from build123d import *

# Parameters (mm, degrees)
SKETCH1_W                     = 935.9
SKETCH1_H                     = 526.4
SKETCH1_R                     = 57.5
BASE_FLANGE1_DEPTH            = 0.7366
EDGE_FLANGE1_STRIP_W          = 4.4196
EDGE_FLANGE1_STRIP_H          = 0.7366
EDGE_FLANGE1_STRIP_CUT_DEPTH  = 935.9
EDGE_FLANGE1_DEPTH            = 935.9
EDGE_FLANGE2_STRIP_W          = 4.4196
EDGE_FLANGE2_STRIP_H          = 0.7366
EDGE_FLANGE2_STRIP_CUT_DEPTH  = 524.9268
EDGE_FLANGE2_DEPTH            = 524.9268
EDGE_FLANGE3_STRIP_W          = 4.4196
EDGE_FLANGE3_STRIP_H          = 0.7366
EDGE_FLANGE3_STRIP_CUT_DEPTH  = 934.4268
EDGE_FLANGE3_DEPTH            = 934.4268
EDGE_FLANGE4_STRIP_W          = 4.4196
EDGE_FLANGE4_STRIP_H          = 0.7366
EDGE_FLANGE4_STRIP_CUT_DEPTH  = 523.4536
EDGE_FLANGE4_DEPTH            = 523.4536
EDGE_FLANGE5_STRIP_W          = 4.4196
EDGE_FLANGE5_STRIP_H          = 0.7366
EDGE_FLANGE5_STRIP_CUT_DEPTH  = 874.0268
EDGE_FLANGE5_RELIEF_W         = 4.7879
EDGE_FLANGE5_RELIEF_H         = 0.3683
EDGE_FLANGE5_RELIEF_CUT_DEPTH = 0.7366
EDGE_FLANGE5_DEPTH            = 874.0268
EDGE_FLANGE6_STRIP_W          = 4.4196
EDGE_FLANGE6_STRIP_H          = 0.7366
EDGE_FLANGE6_STRIP_CUT_DEPTH  = 874.0268
EDGE_FLANGE6_RELIEF_W         = 4.7879
EDGE_FLANGE6_RELIEF_H         = 0.3683
EDGE_FLANGE6_RELIEF_CUT_DEPTH = 0.7366
EDGE_FLANGE6_DEPTH            = 874.0268
EDGE_FLANGE7_STRIP_W          = 4.4196
EDGE_FLANGE7_STRIP_H          = 0.7366
EDGE_FLANGE7_STRIP_CUT_DEPTH  = 523.4536
EDGE_FLANGE7_DEPTH            = 523.4536
EDGE_FLANGE8_STRIP_W          = 4.4196
EDGE_FLANGE8_STRIP_H          = 0.7366
EDGE_FLANGE8_STRIP_CUT_DEPTH  = 523.9902
EDGE_FLANGE8_RELIEF_W         = 4.7879
EDGE_FLANGE8_RELIEF_H         = 0.3683
EDGE_FLANGE8_RELIEF_CUT_DEPTH = 0.7366
EDGE_FLANGE8_DEPTH            = 523.9902


# Sheet-metal steps are written as plain solids
with BuildPart() as part:
    # Sketch1 → Base-Flange1 (new body)
    with BuildSketch(Plane(origin=(0, 0, 0), x_dir=(0, 0, -1), z_dir=(1, 0, 0))):
        Rectangle(SKETCH1_W, SKETCH1_H)
        Circle(SKETCH1_R, mode=Mode.SUBTRACT)
    extrude(amount=-BASE_FLANGE1_DEPTH)

    # Edge-Flange1 strip (across the edge) → Edge-Flange1 strip cut (cut)
    with BuildSketch(Plane(origin=(-0.7366, 263.2, 467.95), x_dir=(0, -1, 0), z_dir=(0, 0, -1))):
        with Locations((-0.7366, -0.3683)):
            Rectangle(EDGE_FLANGE1_STRIP_W, EDGE_FLANGE1_STRIP_H)
    extrude(amount=EDGE_FLANGE1_STRIP_CUT_DEPTH, mode=Mode.SUBTRACT)

    # Edge-Flange1 section (across the edge) → Edge-Flange1 (add)
    with BuildSketch(Plane(origin=(-0.7366, 263.2, 467.95), x_dir=(0, -1, 0), z_dir=(0, 0, -1))):
        with BuildLine():
            Line((0, 0.7366), (0, 29.2634))
            Line((0, 29.2634), (0.7366, 29.2634))
            Line((0.7366, 29.2634), (0.7366, 0.7366))
            ThreePointArc((0.7366, 0.7366), (0.952345145, 0.215745145), (1.4732, 0))
            Line((1.4732, 0), (1.4732, -0.7366))
            ThreePointArc((1.4732, -0.7366), (0.43149029, -0.30510971), (0, 0.7366))
        make_face()
    extrude(amount=EDGE_FLANGE1_DEPTH)

    # Edge-Flange2 strip (across the edge) → Edge-Flange2 strip cut (cut)
    with BuildSketch(Plane(origin=(-0.7366, -263.2, 467.95), x_dir=(0, 0, -1), z_dir=(0, 1, 0))):
        with Locations((-0.7366, -0.3683)):
            Rectangle(EDGE_FLANGE2_STRIP_W, EDGE_FLANGE2_STRIP_H)
    extrude(amount=EDGE_FLANGE2_STRIP_CUT_DEPTH, mode=Mode.SUBTRACT)

    # Edge-Flange2 section (across the edge) → Edge-Flange2 (add)
    with BuildSketch(Plane(origin=(-0.7366, -263.2, 467.95), x_dir=(0, 0, -1), z_dir=(0, 1, 0))):
        with BuildLine():
            Line((0, 0.7366), (0, 29.2634))
            Line((0, 29.2634), (0.7366, 29.2634))
            Line((0.7366, 29.2634), (0.7366, 0.7366))
            ThreePointArc((0.7366, 0.7366), (0.952345145, 0.215745145), (1.4732, 0))
            Line((1.4732, 0), (1.4732, -0.7366))
            ThreePointArc((1.4732, -0.7366), (0.43149029, -0.30510971), (0, 0.7366))
        make_face()
    extrude(amount=EDGE_FLANGE2_DEPTH)

    # Edge-Flange3 strip (across the edge) → Edge-Flange3 strip cut (cut)
    with BuildSketch(Plane(origin=(-0.7366, -263.2, -467.95), x_dir=(0, 1, 0), z_dir=(0, 0, 1))):
        with Locations((-0.7366, -0.3683)):
            Rectangle(EDGE_FLANGE3_STRIP_W, EDGE_FLANGE3_STRIP_H)
    extrude(amount=EDGE_FLANGE3_STRIP_CUT_DEPTH, mode=Mode.SUBTRACT)

    # Edge-Flange3 section (across the edge) → Edge-Flange3 (add)
    with BuildSketch(Plane(origin=(-0.7366, -263.2, -467.95), x_dir=(0, 1, 0), z_dir=(0, 0, 1))):
        with BuildLine():
            Line((0, 0.7366), (0, 29.2634))
            Line((0, 29.2634), (0.7366, 29.2634))
            Line((0.7366, 29.2634), (0.7366, 0.7366))
            ThreePointArc((0.7366, 0.7366), (0.952345145, 0.215745145), (1.4732, 0))
            Line((1.4732, 0), (1.4732, -0.7366))
            ThreePointArc((1.4732, -0.7366), (0.43149029, -0.30510971), (0, 0.7366))
        make_face()
    extrude(amount=EDGE_FLANGE3_DEPTH)

    # Edge-Flange4 strip (across the edge) → Edge-Flange4 strip cut (cut)
    with BuildSketch(Plane(origin=(-0.7366, 261.7268, -467.95), x_dir=(0, 0, 1), z_dir=(0, -1, 0))):
        with Locations((-0.7366, -0.3683)):
            Rectangle(EDGE_FLANGE4_STRIP_W, EDGE_FLANGE4_STRIP_H)
    extrude(amount=EDGE_FLANGE4_STRIP_CUT_DEPTH, mode=Mode.SUBTRACT)

    # Edge-Flange4 section (across the edge) → Edge-Flange4 (add)
    with BuildSketch(Plane(origin=(-0.7366, 261.7268, -467.95), x_dir=(0, 0, 1), z_dir=(0, -1, 0))):
        with BuildLine():
            Line((0, 0.7366), (0, 29.2634))
            Line((0, 29.2634), (0.7366, 29.2634))
            Line((0.7366, 29.2634), (0.7366, 0.7366))
            ThreePointArc((0.7366, 0.7366), (0.952345145, 0.215745145), (1.4732, 0))
            Line((1.4732, 0), (1.4732, -0.7366))
            ThreePointArc((1.4732, -0.7366), (0.43149029, -0.30510971), (0, 0.7366))
        make_face()
    extrude(amount=EDGE_FLANGE4_DEPTH)

    # Edge-Flange5 strip (across the edge) → Edge-Flange5 strip cut (cut)
    with BuildSketch(Plane(origin=(-30, 262.4634, 437.0134), x_dir=(1, 0, 0), z_dir=(0, 0, -1))):
        with Locations((-0.7366, -0.3683)):
            Rectangle(EDGE_FLANGE5_STRIP_W, EDGE_FLANGE5_STRIP_H)
    extrude(amount=EDGE_FLANGE5_STRIP_CUT_DEPTH, mode=Mode.SUBTRACT)

    # Edge-Flange5 relief (on the sheet) → Edge-Flange5 relief cut (cut)
    with BuildSketch(Plane(origin=(-28.5268, 262.4634, 437.0134), x_dir=(1, 0, 0), z_dir=(0, -1, 0))):
        with Locations((-2.02565, 0.18415)):
            Rectangle(EDGE_FLANGE5_RELIEF_W, EDGE_FLANGE5_RELIEF_H)
        with Locations((-2.02565, -874.21095)):
            Rectangle(EDGE_FLANGE5_RELIEF_W, EDGE_FLANGE5_RELIEF_H)
    extrude(amount=-EDGE_FLANGE5_RELIEF_CUT_DEPTH, mode=Mode.SUBTRACT)

    # Edge-Flange5 section (across the edge) → Edge-Flange5 (add)
    with BuildSketch(Plane(origin=(-30, 262.4634, 437.0134), x_dir=(1, 0, 0), z_dir=(0, 0, -1))):
        with BuildLine():
            Line((0, 0.7366), (0, 29.2634))
            Line((0, 29.2634), (0.7366, 29.2634))
            Line((0.7366, 29.2634), (0.7366, 0.7366))
            ThreePointArc((0.7366, 0.7366), (0.952345145, 0.215745145), (1.4732, 0))
            Line((1.4732, 0), (1.4732, -0.7366))
            ThreePointArc((1.4732, -0.7366), (0.43149029, -0.30510971), (0, 0.7366))
        make_face()
    extrude(amount=EDGE_FLANGE5_DEPTH)

    # Edge-Flange6 strip (across the edge) → Edge-Flange6 strip cut (cut)
    with BuildSketch(Plane(origin=(-30, -262.4634, -437.0134), x_dir=(1, 0, 0), z_dir=(0, 0, 1))):
        with Locations((-0.7366, -0.3683)):
            Rectangle(EDGE_FLANGE6_STRIP_W, EDGE_FLANGE6_STRIP_H)
    extrude(amount=EDGE_FLANGE6_STRIP_CUT_DEPTH, mode=Mode.SUBTRACT)

    # Edge-Flange6 relief (on the sheet) → Edge-Flange6 relief cut (cut)
    with BuildSketch(Plane(origin=(-28.5268, -262.4634, -437.0134), x_dir=(1, 0, 0), z_dir=(0, 1, 0))):
        with Locations((-2.02565, 0.18415)):
            Rectangle(EDGE_FLANGE6_RELIEF_W, EDGE_FLANGE6_RELIEF_H)
        with Locations((-2.02565, -874.21095)):
            Rectangle(EDGE_FLANGE6_RELIEF_W, EDGE_FLANGE6_RELIEF_H)
    extrude(amount=-EDGE_FLANGE6_RELIEF_CUT_DEPTH, mode=Mode.SUBTRACT)

    # Edge-Flange6 section (across the edge) → Edge-Flange6 (add)
    with BuildSketch(Plane(origin=(-30, -262.4634, -437.0134), x_dir=(1, 0, 0), z_dir=(0, 0, 1))):
        with BuildLine():
            Line((0, 0.7366), (0, 29.2634))
            Line((0, 29.2634), (0.7366, 29.2634))
            Line((0.7366, 29.2634), (0.7366, 0.7366))
            ThreePointArc((0.7366, 0.7366), (0.952345145, 0.215745145), (1.4732, 0))
            Line((1.4732, 0), (1.4732, -0.7366))
            ThreePointArc((1.4732, -0.7366), (0.43149029, -0.30510971), (0, 0.7366))
        make_face()
    extrude(amount=EDGE_FLANGE6_DEPTH)

    # Edge-Flange7 strip (across the edge) → Edge-Flange7 strip cut (cut)
    with BuildSketch(Plane(origin=(-30, 261.7268, -467.2134), x_dir=(1, 0, 0), z_dir=(0, -1, 0))):
        with Locations((-0.7366, -0.3683)):
            Rectangle(EDGE_FLANGE7_STRIP_W, EDGE_FLANGE7_STRIP_H)
    extrude(amount=EDGE_FLANGE7_STRIP_CUT_DEPTH, mode=Mode.SUBTRACT)

    # Edge-Flange7 section (across the edge) → Edge-Flange7 (add)
    with BuildSketch(Plane(origin=(-30, 261.7268, -467.2134), x_dir=(1, 0, 0), z_dir=(0, -1, 0))):
        with BuildLine():
            Line((0, 0.7366), (0, 29.2634))
            Line((0, 29.2634), (0.7366, 29.2634))
            Line((0.7366, 29.2634), (0.7366, 0.7366))
            ThreePointArc((0.7366, 0.7366), (0.952345145, 0.215745145), (1.4732, 0))
            Line((1.4732, 0), (1.4732, -0.7366))
            ThreePointArc((1.4732, -0.7366), (0.43149029, -0.30510971), (0, 0.7366))
        make_face()
    extrude(amount=EDGE_FLANGE7_DEPTH)

    # Edge-Flange8 strip (across the edge) → Edge-Flange8 strip cut (cut)
    with BuildSketch(Plane(origin=(-30, -262.2634, 467.2134), x_dir=(1, 0, 0), z_dir=(0, 1, 0))):
        with Locations((-0.7366, -0.3683)):
            Rectangle(EDGE_FLANGE8_STRIP_W, EDGE_FLANGE8_STRIP_H)
    extrude(amount=EDGE_FLANGE8_STRIP_CUT_DEPTH, mode=Mode.SUBTRACT)

    # Edge-Flange8 relief (on the sheet) → Edge-Flange8 relief cut (cut)
    with BuildSketch(Plane(origin=(-28.5268, -262.2634, 467.2134), x_dir=(1, 0, 0), z_dir=(0, 0, -1))):
        with Locations((-2.02565, 0.18415)):
            Rectangle(EDGE_FLANGE8_RELIEF_W, EDGE_FLANGE8_RELIEF_H)
    extrude(amount=-EDGE_FLANGE8_RELIEF_CUT_DEPTH, mode=Mode.SUBTRACT)

    # Edge-Flange8 section (across the edge) → Edge-Flange8 (add)
    with BuildSketch(Plane(origin=(-30, -262.2634, 467.2134), x_dir=(1, 0, 0), z_dir=(0, 1, 0))):
        with BuildLine():
            Line((0, 0.7366), (0, 29.2634))
            Line((0, 29.2634), (0.7366, 29.2634))
            Line((0.7366, 29.2634), (0.7366, 0.7366))
            ThreePointArc((0.7366, 0.7366), (0.952345145, 0.215745145), (1.4732, 0))
            Line((1.4732, 0), (1.4732, -0.7366))
            ThreePointArc((1.4732, -0.7366), (0.43149029, -0.30510971), (0, 0.7366))
        make_face()
    extrude(amount=EDGE_FLANGE8_DEPTH)


solid = part.part
Input: part model. Units: mm. Frame: model coordinates. A direction names the side the tool comes from. Give positions to 0.01 mm unless a question says otherwise; leave off trailing zeros. Loops run counter-clockwise (first coordinate to the right, second up) from the corner with the lowest first, then second, coordinate; pieces in that order, holes last. Notation, with made-up numbers: M 68,58 L 73,58 A24 ccw 73,91 Z; hole C 9,-25 d7. An arc over 180 degrees is marked long. Use one line per item in the form item = value.
1. Line query: L1, parallel to Z at x = -7.5, y = 9; L2, parallel to Y at x = -4.5, z = 261; L3, parallel to X at y = 242, z = 250.5. Output: solid intervals per line, ascending.
Numbers:
L1 = -467.95 to -467.21, 467.21 to 467.95
L2 = -263.2 to -262.46, 262.46 to 263.2
L3 = -30 to -29.26, -0.74 to 0
2. Reachability of faces 1 (the face through (-29.263, 4, -452)), 2 (the face through (-30, -4, 452)), 3 (the face through (-16, -4, 467.213)) from +Z, -Z, +X, -X, +Y, -Y: full face, straight path, thin tool, end or side. Return the list, or none.
Numbers:
face_1 = none
face_2 = +Z, -Z, -X, +Y, -Y
face_3 = -Y
3. Section query D-D, the plane y = 174.5. Return the cut outline in (x, z).
Numbers:
outline = M -30,-466.48 A1.47 ccw -28.53,-467.95 L -1.47,-467.95 A1.47 ccw 0,-466.48 L 0,466.48 A1.47 ccw -1.47,467.95 L -28.53,467.95 A1.47 ccw -30,466.48 L -30,437.95 L -29.26,437.95 L -29.26,466.48 A0.74 cw -28.53,467.21 L -1.47,467.21 A0.74 cw -0.74,466.48 L -0.74,-466.48 A0.74 cw -1.47,-467.21 L -28.53,-467.21 A0.74 cw -29.26,-466.48 L -29.26,-437.95 L -30,-437.95 Z
4. First-contact query: pin 1 (4 mm diameter, centred on y = 141.5, z = 220.5, fed in from -X); pin 2 (0.8 mm diameter, centred on x = -0.5, z = -467.5, fed in from -Y). Flat tips, straight axial feed; report the tip coordinate or a pass-through.
Numbers:
pin_1 = -0.74
pin_2 = -263.08
5. Section query A-A, the plane y = 0. Return the cut outline in (x, z), and give its area (4 significant figures).
Numbers:
outline = M -30,-466.48 A1.47 ccw -28.53,-467.95 L -1.47,-467.95 A1.47 ccw 0,-466.48 L 0,-57.5 L -0.74,-57.5 L -0.74,-466.48 A0.74 cw -1.47,-467.21 L -28.53,-467.21 A0.74 cw -29.26,-466.48 L -29.26,-437.95 L -30,-437.95 Z; M -30,437.95 L -29.26,437.95 L -29.26,466.48 A0.74 cw -28.53,467.21 L -1.47,467.21 A0.74 cw -0.74,466.48 L -0.74,57.5 L 0,57.5 L 0,466.48 A1.47 ccw -1.47,467.95 L -28.53,467.95 A1.47 ccw -30,466.48 Z
area = 689.5 mm²
6. Section query B-B, the plane x = -9. Return the cut outline in (y, z), and give its area (3 significant figures).
Numbers:
outline = M -263.2,-467.95 L -262.46,-467.95 L -262.46,466.48 L -263.2,466.48 Z; M -263.2,467.21 L 261.73,467.21 L 261.73,467.95 L -263.2,467.95 Z; M -261.73,-467.95 L 261.73,-467.95 L 261.73,-467.21 L -261.73,-467.21 Z; M 262.46,-467.95 L 263.2,-467.95 L 263.2,467.95 L 262.46,467.95 Z
area = 2,150 mm²
7. Section query C-C, the plane z = 0. Return the cut outline in (x, y), and give its area (3 significant figures).
Numbers:
outline = M -30,-261.73 A1.47 ccw -28.53,-263.2 L -1.47,-263.2 A1.47 ccw 0,-261.73 L 0,-57.5 L -0.74,-57.5 L -0.74,-261.73 A0.74 cw -1.47,-262.46 L -28.53,-262.46 A0.74 cw -29.26,-261.73 L -29.26,-233.2 L -30,-233.2 Z; M -30,233.2 L -29.26,233.2 L -29.26,261.73 A0.74 cw -28.53,262.46 L -1.47,262.46 A0.74 cw -0.74,261.73 L -0.74,57.5 L 0,57.5 L 0,261.73 A1.47 ccw -1.47,263.2 L -28.53,263.2 A1.47 ccw -30,261.73 Z
area = 388 mm²
8. Pull-direction query (Y, two-part tool) for faces 4 (the face through (-16, 263.2, 7)), 5 (the face through (-30, 248, 6)), 6 (the face through (-15, 4, -467.213)), 7 (the face through (-16, -263.2, -7)); classes: released by +Y, released by -Y, zero draft, split by the parting line, or undercut.
Numbers:
face_4 = released by +Y
face_5 = zero draft
face_6 = undercut
face_7 = released by -Y
